Build history of the part. All positions in model axes, mm. A direction names the side the tool comes from. Round coordinates to 2 decimals unless told otherwise and drop trailing zeros. Loops run counter-clockwise (first coordinate to the right, second up) from the corner with the lowest first, then second, coordinate; pieces in that order, holes last. Notation, with made-up numbers: (-18.75, 86) -> (11.25, 86) arc R32 ccw to (11.25, 116) -> close; hole circle Ø7 at (-11, 88.25). An arc over 180 degrees is marked (long way). Put each result on its own line as item: value. Start each with the question number.
```python
from build123d import *

# Parameters (mm, degrees)
F3_DEPTH = 25
F4_DEPTH = 25
F5_DEPTH = 25


with BuildPart() as f3:
    # F0 (on Front) → F3 (new body, symmetric)
    with BuildSketch(Plane.XZ):
        Polygon((-7.5, 25), (-25, 25), (-25, 10.391577), (-25, -13.939915), (-25, -25), (-7.5, -25), (-7.5, -5.072788), (7.5, -5.072788), (7.5, -25), (25, -25), (25, -13.939915), (25, 10.391577), (25, 25), (7.5, 25), (7.5, 4.447581), (-7.5, 4.447581), align=None)
    extrude(amount=F3_DEPTH, both=True)

    # F2 (on Right) → F4 (intersect, symmetric)
    with BuildSketch(Plane.YZ):
        Polygon((-25, -25), (-14.815953, -25), (-14.815953, -8.320933), (-5.655421, -4.472235), (11.595094, -25), (25, -25), (4.989232, 0), (25, 8.407306), (25, 25), (-14.815953, 0), (-14.815953, 25), (-25, 25), align=None)
    extrude(amount=F4_DEPTH, both=True, mode=Mode.INTERSECT)

    # F1 (on Top) → F5 (intersect, symmetric)
    with BuildSketch(Plane.XY):
        Polygon((-12.632664, 25), (-25, -25), (-9.547958, -25), (-5.475463, -8.535276), (0, -17.231597), (4.751956, -8.469481), (9.423391, -25), (25, -24.961657), (10.881108, 25), (0, 4.936364), align=None)
    extrude(amount=F5_DEPTH, both=True, mode=Mode.INTERSECT)


solid = f3.part
```
Item 1: Pull direction X, two halves, no side cores. Call faces 1 (the face through (7.5, -16, -13)), 2 (the face through (-12, 17, -25)): +X half, -X half, draft (parallel to the pull), parting line (faces both ways), or undercut.
Item 2: Cut at B-B on y = 7. Write the cut outline in (x, z), then the cut area to 3 significant figures.
Item 3: Cut at C-C on z = -6.5. Write the cut outline in (x, y), then the cut area to 3 significant figures.
Item 4: Drop flat-ended pins along their axis: pin 1 (3.5 mm diameter, centred on x = -3.5, y = -10.5, fed in from -Z); pin 2 (0.8 mm diameter, centred on x = 7, y = -17.5, fed in from +Z); pin 3 (6 mm diameter, centred on y = 0.5, z = -12.5, fed in from +X). Give the stop position or say it passes through.
Item 5: Wall check: line 1 (X direction, y = -17.5, z = -14); line 2 (Y direction, x = 19, z = -20); line 3 (Y direction, x = -14, z = 6). Give the ranges that are in metal, low to high. Write a range as from..to.
Item 6: 3-axis set-ups, long thin cutter, end or side, ignore diameter. For faces 3 (the face through (8.463, 20.541, -22.782)), 4 (the face through (-10.63, 12.63, 3.21)), 5 (the face through (7.5, -17, 15)), 6 (the face through (0, -10, -5.073)): which of +Z, -Z, +X, -X, +Y, -Y reach the whole face in a straight line?
Item 7: Cut at A-A on y = -19.5. Write the cut outline in (x, z).
Item 8: Cut at D-D on x = 3. Write the cut outline in (y, z), then the cut area to 3 significant figures.
Ans:
1. face 1: undercut
1. face 2: draft
2. outline: (-17.08, -19.53) -> (-7.5, -19.53) -> (-7.5, -5.07) -> (-1.3, -5.07) -> (-1.3, -2.51) -> (-17.08, -2.51) -> close; (-17.08, 0.84) -> (-1.3, 0.84) -> (-1.3, 4.45) -> (-7.5, 4.45) -> (-7.5, 13.7) -> (-17.08, 13.7) -> close; (1.12, -5.07) -> (7.5, -5.07) -> (7.5, -19.53) -> (15.97, -19.53) -> (15.97, -2.51) -> (1.12, -2.51) -> close; (1.12, 0.84) -> (15.97, 0.84) -> (15.97, 13.7) -> (7.5, 13.7) -> (7.5, 4.45) -> (1.12, 4.45) -> close
2. area: 617 mm2
3. outline: (-25, -25) -> (-9.55, -25) -> (-7.5, -16.72) -> (-7.5, -10.48) -> (-21.41, -10.48) -> close; (-19.79, -3.95) -> (-7.5, -3.95) -> (-7.5, 10.19) -> (-16.3, 10.19) -> close; (7.5, -18.19) -> (9.42, -25) -> (25, -24.96) -> (20.91, -10.48) -> (7.5, -10.48) -> close; (7.5, -3.95) -> (19.06, -3.95) -> (15.07, 10.19) -> (7.5, 10.19) -> close
3. area: 722 mm2
4. pin 1: stops at z = -5.07
4. pin 2: stops at z = 4.45
4. pin 3: stops at x = 18.25
5. line 1: x = -23.14..-7.69, 7.5..22.89
5. line 2: y = -24.98..-14.82
5. line 3: y = -25..-14.82, -5.26..19.27
6. face 3: +Z, -Z, +Y
6. face 4: +X, -X, +Y
6. face 5: +Z, +Y, -Y
6. face 6: -Z, +Y, -Y
7. outline: (-23.64, -25) -> (-8.19, -25) -> (-8.19, 25) -> (-23.64, 25) -> close; (7.87, -25) -> (23.46, -25) -> (23.46, 25) -> (7.87, 25) -> close
8. outline: (-11.7, -5.07) -> (-7.08, -5.07) -> (-5.66, -4.47) -> (-5.15, -5.07) -> (9.05, -5.07) -> (4.99, 0) -> (10.47, 2.3) -> (10.47, 4.45) -> (-7.73, 4.45) -> (-11.7, 1.96) -> close
8. area: 182 mm2
